```python
from build123d import *

# Parameters (mm, degrees)
F0_R          = 12.7
F0_R_2        = 3.175
F1_DEPTH      = 31.75
F3_DEPTH      = 12.7
F3_DEPTH_BACK = 12.7
F4_R          = 3.048
F5_R          = 6.35
F6_R          = 3.175
F7_DEPTH      = 44.17668
F8_R          = 3.175
F9_DEPTH      = 44.17568
F10_R         = 3.175
F11_DEPTH     = 3.175
F12_R         = 1.524


with BuildPart() as f1:
    # F0 (on Front) → F1 (new body)
    with BuildSketch(Plane.XZ):
        Circle(F0_R)
        Circle(F0_R_2, mode=Mode.SUBTRACT)
    extrude(amount=F1_DEPTH)



with BuildPart() as f3:
    # F2 (on Right) → F3 (new body, two sides)
    with BuildSketch(Plane.YZ) as f3_sk:
        Polygon((-34.925, -20.6375), (-34.925, 9.525), (-37.96284, 9.525), (-37.96284, -23.8125), (6.21284, -23.8125), (6.21284, 9.525), (3.175, 9.525), (3.175, -20.6375), align=None)
    extrude(amount=F3_DEPTH)
    extrude(f3_sk.sketch, amount=-F3_DEPTH_BACK)

    # F4
    f4_edges = [f3.edges().sort_by_distance(p)[0] for p in [
        (0, -37.96284, -23.8125),
        (0, -34.925, -20.6375),
        (0, 3.175, -20.6375),
        (0, 6.21284, -23.8125),
    ]]
    fillet(f4_edges, radius=F4_R)

    # F5
    f5_edges = [f3.edges().sort_by_distance(p)[0] for p in [
        (12.7, -36.44392, 9.525),
        (-12.7, -36.44392, 9.525),
        (-12.7, 4.69392, 9.525),
        (12.7, 4.69392, 9.525),
    ]]
    fillet(f5_edges, radius=F5_R)

    # F6 (on face) → F7 (cut, through all)
    with BuildSketch(Plane.XZ.offset(37.96284)):
        Circle(F6_R)
    extrude(amount=-F7_DEPTH, mode=Mode.SUBTRACT)


with BuildPart() as f1_1:
    add(f1.part)

    add(f3.part)  # F9 merges F3
    # F8 (on face) → F9 (join, through all)
    with BuildSketch(Plane.XZ.offset(37.96284)):
        Circle(F8_R)
    extrude(amount=-F9_DEPTH)

    # F10 (on face) → F11 (cut, through all)
    with BuildSketch(Plane(origin=(0, 0, -23.8125), x_dir=(1, 0, 0), z_dir=(0, 0, -1))):
        with Locations((0, 15.875)):
            Circle(F10_R)
    extrude(amount=-F11_DEPTH, mode=Mode.SUBTRACT)

    # F12
    f12_edges = [f1_1.edges().sort_by_distance(p)[0] for p in [
        (-12.7, -31.75, 0),
        (-12.7, 0, 0),
    ]]
    fillet(f12_edges, radius=F12_R)


solid = f1_1.part
```
Work out the finished part from the listing and answer in its coordinate system (mm). A direction names the side the tool comes from. Coordinates: 2 decimals unless noted, no trailing zeros. Order: outer loops, then holes, each group sorted by start corner. A loop starts at its lowest first (then second) coordinate and runs counter-clockwise, first axis right, second up. Notation, with made-up numbers: (48, 30) - (82, 30) arc R20 ccw to (82, 38) - close; hole circle Ø2 at (49, 49). An arc over 180 degrees is marked (long way). Answer as a JSON object with one key per item and string values.
1. Find section D-D on z = 0. Determine the outline of the cut face in (x, y) (3 decimals).
Output values:
{"outline": "(-12.7, -37.963) - (12.7, -37.963) - (12.7, -34.925) - (3.175, -34.925) - (3.175, -31.75) - (11.176, -31.75) arc R1.524 ccw to (12.7, -30.226) - (12.7, -1.524) arc R1.524 ccw to (11.176, 0) - (3.175, 0) - (3.175, 3.175) - (12.7, 3.175) - (12.7, 6.213) - (-12.7, 6.213) - (-12.7, 3.175) - (-3.175, 3.175) - (-3.175, 0) - (-11.176, 0) arc R1.524 ccw to (-12.7, -1.524) - (-12.7, -30.226) arc R1.524 ccw to (-11.176, -31.75) - (-3.175, -31.75) - (-3.175, -34.925) - (-12.7, -34.925) - close"}
2. Find section B-B on z = -18.5. Determine the outline of the cut face in (x, y).
Output values:
{"outline": "(-12.7, -37.96) - (12.7, -37.96) - (12.7, -34.79) - (-12.7, -34.79) - close; (-12.7, 3.04) - (12.7, 3.04) - (12.7, 6.21) - (-12.7, 6.21) - close"}
3. The mould has two halves that part along Y. Classify faces 1 (the face through (0, -37.963, -5)), 2 (the face through (-10.889, -36.465, 7.615)), 3 (the face through (2, 0, 3)): +Y half, -Y half, draft (parallel to the pull), parting line (faces both ways), or undercut.
Output values:
{"face 1": "-Y half", "face 2": "draft", "face 3": "undercut"}
4. A tool of negligible diameter and unlimited length cuts with its end or side. For faces 4 (the face through (-0.69, -33.36, -3.1)), 5 (the face through (-10.889, 4.673, 7.615)), 6 (the face through (10.79, -36.465, 7.714)), 7 (the face through (-0.413, -19.023, -22.247)), 8 (the face through (0.2, -19.2, -20.638)), from which of +Z, -Z, +X, -X, +Y, -Y can it reach the whole face along a straight path? Write none if from no direction.
Output values:
{"face 4": "none", "face 5": "+Z, -X, +Y", "face 6": "+Z, +X, -Y", "face 7": "-Z", "face 8": "+X, -X"}
5. Consider line 1 (Y direction, x = -2.5, z = -6.5) (3 decimals); line 2 (Y direction, x = 6.75, z = 9) (3 decimals); line 3 (Z direction, x = 10.5, y = -22). Determine where each line is inside the solid, lowest interval first.
Output values:
{"line 1": "y = -37.963 to -34.925, -31.75 to 0, 3.175 to 6.213", "line 2": "y = -37.963 to -34.925, -31.748 to -0.002, 3.175 to 6.213", "line 3": "z = -23.81 to -20.64, -7.14 to 7.14"}
6. Find section A-A on y = -4.5. Determine the outline of the cut face in (x, z), plus the area to 3 significant figures.
Output values:
{"outline": "(-12.7, -23.81) - (12.7, -23.81) - (12.7, -20.64) - (-12.7, -20.64) - close; circle Ø25.4 at (0, 0)", "area": "587 mm²"}
7. Each of these flat-tipped pins is pushed along its axis until it touches: P1, Ø8, axis at x = 9, y = -15.5, coming from the +Z side; P2, Ø10, axis at x = 6, y = -28, coming from the +Z side; P3, Ø2.5, axis at x = 2, y = -36, coming from the +Z side (3 decimals). Where does it stop, or does it pass through?
Output values:
{"P1": "stops at z = 11.67", "P2": "stops at z = 12.66", "P3": "stops at z = 9.525"}
